The listing builds one solid part. Answer for the finished solid, in the listing's coordinates (mm). Face numbers are marked on the shaded views. Coordinates: 2 decimals unless noted, no trailing zeros. Order: outer loops, then holes, each group sorted by start corner. A loop starts at its lowest first (then second) coordinate and runs counter-clockwise, first axis right, second up. Notation, with made-up numbers: (10.25, -34) -> (48.25, -34) arc R17 cw to (48.25, -25) -> close; hole circle Ø1 at (-31, 7). An arc over 180 degrees is marked (long way). One line per question, with ' | ' between items.
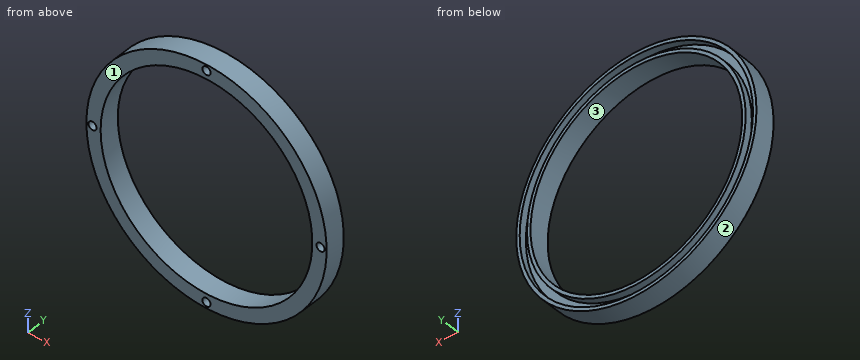
Autodesk Inventor part; units mm, degrees
ref_plane "Work Plane1" through (0, 4.1, 0) normal (0, 1, 0) x (-1, 0, 0)
ref_plane "YZ Plane" through (0, 0, 0) normal (1, 0, 0) x (0, 1, 0)
ref_plane "XY Plane" through (0, 0, 0) normal (0, 0, 1) x (1, 0, 0)
sketch "Sketch14" plane through (0, 0, 0) normal (0, 1, 0) x (-1, 0, 0)
  circle A0 centre (0, 0) radius 26
  circle A1 centre (0, 0) radius 29.5
  dimension "d122" = 52
  dimension "d123" = 59
extrude "Extrusion3" add sketch "Sketch14" along normal blind 5
sketch "Sketch15" plane through (0, 5, 0) normal (0, 1, 0) x (1, 0, 0)
  circle A0 centre (0, 0) radius 26.85
  circle A1 centre (0, 0) radius 28.65
  dimension "d126" = 53.7
  dimension "d127" = 57.3
extrude "Extrusion4" cut sketch "Sketch15" against normal blind 1.8
ref_plane "Work Plane1" through (0, 4.1, 0) normal (0, 1, 0) x (-1, 0, 0)
sketch "Sketch16" plane through (0, 0, 0) normal (0, -1, 0) x (1, 0, 0)
  circle A0 centre (28, 0) radius 1
  point P0 (0, 0)
  dimension "d131" = 2
  dimension "d132" = 28
hole "Hole12" at (28, 0, 0) direction (0, 1, 0) diameter 2 depth 2
sketch "Sketch17" plane through (0, 0, 0) normal (0, -1, 0) x (1, 0, 0)
  circle A0 centre (0, -28) radius 1
  point P0 (0, 0)
  dimension "d140" = 2
  dimension "d141" = 28
hole "Hole13" at (0, 0, -28) direction (0, 1, 0) diameter 2 depth 2
sketch "Sketch18" plane through (0, 0, 0) normal (0, -1, 0) x (1, 0, 0)
  circle A0 centre (0, 28) radius 1
  point P0 (0, 0)
  dimension "d149" = 2
  dimension "d150" = 28
hole "Hole14" at (0, 0, 28) direction (0, 1, 0) diameter 2 depth 2
sketch "Sketch19" plane through (0, 0, 0) normal (0, -1, 0) x (1, 0, 0)
  circle A0 centre (-28, 0) radius 1
  point P0 (0, 0)
  dimension "d158" = 2
  dimension "d159" = 28
hole "Hole15" at (-28, 0, 0) direction (0, 1, 0) diameter 2 depth 2
thread "Thread5"
thread "Thread6"
thread "Thread7"
thread "Thread8"
properties part number "Cap"
Item 1: Section C-C, the plane z = 19 is taken. Give the vertices of the cut face in (x, y), plus the area to 3 significant figures.
Computed values:
outline: (-22.57, 0) -> (-17.75, 0) -> (-17.75, 5) -> (-18.97, 5) -> (-18.97, 3.2) -> (-21.44, 3.2) -> (-21.44, 5) -> (-22.57, 5) -> close; (17.75, 0) -> (22.57, 0) -> (22.57, 5) -> (21.44, 5) -> (21.44, 3.2) -> (18.97, 3.2) -> (18.97, 5) -> (17.75, 5) -> close | area: 39.3 mm^2
Item 2: Each of these flat-tipped pins is pushed along its axis until it touches: pin 1 Ø1 at (x, z) = (0, 28) entering from -Y; pin 2 Ø2 at (x, y) = (23, 3.5) entering from +Z; pin 3 Ø1 at (y, z) = (2, 21) entering from -X. Where does it stop, or does it pass through?
Computed values:
pin 1: stops at y = 2 | pin 2: stops at z = 19.65 | pin 3: stops at x = -21.21
Item 3: Find the intervals of material crossed by L1, parallel to Z at x = 0, y = 4.4; L2, parallel to Z at x = -11, y = 4.65; L3, parallel to X at y = 4.45, z = -3, in increasing order.
Computed values:
L1: z = -29.5 to -28.65, -26.85 to -26, 26 to 26.85, 28.65 to 29.5 | L2: z = -27.37 to -26.45, -24.49 to -23.56, 23.56 to 24.49, 26.45 to 27.37 | L3: x = -29.35 to -28.49, -26.68 to -25.83, 25.83 to 26.68, 28.49 to 29.35
Item 4: Determine the mould class of the marked faces 1, 2 and 3 for opening direction Z: pulls with the +Z half, pulls with the -Z half, needs draft (parallel to the pull), parting line crosses it, or undercut.
Computed values:
face 1: needs draft | face 2: parting line crosses it | face 3: undercut
Item 5: Section B-B, the plane z = -19.5 is taken. Give the vertices of the cut face in (x, y), plus the area to 3 significant figures.
Computed values:
outline: (-22.14, 0) -> (-17.2, 0) -> (-17.2, 5) -> (-18.46, 5) -> (-18.46, 3.2) -> (-20.99, 3.2) -> (-20.99, 5) -> (-22.14, 5) -> close; (17.2, 0) -> (22.14, 0) -> (22.14, 5) -> (20.99, 5) -> (20.99, 3.2) -> (18.46, 3.2) -> (18.46, 5) -> (17.2, 5) -> close | area: 40.3 mm^2
Item 6: Section A-A, the plane x = 0 is taken. Give the vertices of the cut face in (y, z).
Computed values:
outline: (0, -29.5) -> (5, -29.5) -> (5, -28.65) -> (3.2, -28.65) -> (3.2, -26.85) -> (5, -26.85) -> (5, -26) -> (0, -26) -> (0, -27) -> (2, -27) -> (2, -29) -> (0, -29) -> close; (0, 26) -> (5, 26) -> (5, 26.85) -> (3.2, 26.85) -> (3.2, 28.65) -> (5, 28.65) -> (5, 29.5) -> (0, 29.5) -> (0, 29) -> (2, 29) -> (2, 27) -> (0, 27) -> close
